The model under review builds one solid part; all positions refer to its coordinate system, in mm. Round coordinates to 2 decimals unless told otherwise and drop trailing zeros. Write each loop counter-clockwise with the first axis right and the second up, starting at its lowest first coordinate (ties: lowest second). Pieces come first, ordered by that corner, then holes. Notation, with made-up numbers: (48, -2.75) - (74, -2.75) arc R27 cw to (74, 21.25) - close; hole circle Ø4 at (46.25, -12). An arc over 180 degrees is marked (long way). Use one line per item in the form item = value.
from build123d import *

# Parameters (mm, degrees)
BOSS_EXTRUDE1_DEPTH = 2590.8
CUT_EXTRUDE1_DEPTH  = 2591.8
BOSS_EXTRUDE2_DEPTH = 2590.8
FILLET1_R           = 0.508


with BuildPart() as part:
    # Sketch1 → Boss-Extrude1 (new body)
    with BuildSketch(Plane(origin=(0, 0, 0), x_dir=(1, 0, 0), z_dir=(0, 1, 0))):
        with BuildLine():
            Line((101.58476, 5.338063609), (101.58476, 6.354063609))
            ThreePointArc((101.58476, 6.354063609), (50.79238, 19.05), (0, 6.354063609))
            Line((0, 6.354063609), (0, 5.338063609))
            Line((0, 5.338063609), (1.338554634, 5.338063609))
            ThreePointArc((1.338554634, 5.338063609), (45.188812602, 17.378377427), (90.062082389, 10.016044959))
            ThreePointArc((90.062082389, 10.016044959), (91.218156641, 9.549225792), (92.368682931, 9.068895628))
            ThreePointArc((92.368682931, 9.068895628), (96.251044015, 7.328911154), (100.06076, 5.435148318))
            Line((100.06076, 5.435148318), (100.06076, 4.322063609))
            ThreePointArc((100.06076, 4.322063609), (100.209549755, 3.962853364), (100.56876, 3.814063609))
            Line((100.56876, 3.814063609), (100.82276, 3.814063609))
            Line((100.82276, 3.814063609), (101.58476, 5.338063609))
        make_face()
    extrude(amount=BOSS_EXTRUDE1_DEPTH)

    # Sketch3 → Cut-Extrude1 (cut, through all)
    with BuildSketch(Plane(origin=(0, 2590.8, 0), x_dir=(1, 0, 0), z_dir=(0, 1, 0))):
        Polygon((100.06076, 2.923708758), (101.58476, 2.923708758), (101.58476, 5.592063609), (100.06076, 5.435148318), align=None)
        Polygon((0, 5.592063609), (0.4067845, 4.474432381), (0, 4.474432381), align=None)
    extrude(amount=-CUT_EXTRUDE1_DEPTH, mode=Mode.SUBTRACT)

    # Sketch2 → Boss-Extrude2 (add)
    with BuildSketch(Plane(origin=(0, 2590.8, 0), x_dir=(1, 0, 0), z_dir=(0, 1, 0))):
        with BuildLine():
            Line((101.238078351, 4.639563606), (101.58476, 5.592063609))
            Line((101.58476, 5.592063609), (97.711183428, 6.625490634))
            ThreePointArc((97.711183428, 6.625490634), (97.924124129, 6.275131553), (97.695976798, 5.934479203))
            ThreePointArc((97.695976798, 5.934479203), (96.254692814, 2.421137976), (99.718733273, 0.865088556))
            ThreePointArc((99.718733273, 0.865088556), (99.858345852, 0.953692868), (99.947271519, 1.093100982))
            Line((99.947271519, 1.093100982), (100.173716674, 1.715253931))
            ThreePointArc((100.173716674, 1.715253931), (100.127790714, 2.064096228), (99.815693785, 2.226563606))
            Line((99.815693785, 2.226563606), (98.79076, 2.226563606))
            ThreePointArc((98.79076, 2.226563606), (97.58426, 3.433063606), (98.79076, 4.639563606))
            Line((98.79076, 4.639563606), (101.238078351, 4.639563606))
        make_face()
        with BuildLine():
            ThreePointArc((1.769066215, 2.226563606), (1.456969286, 2.064096228), (1.411043326, 1.715253931))
            Line((1.411043326, 1.715253931), (1.637488481, 1.093100982))
            ThreePointArc((1.637488481, 1.093100982), (1.726414148, 0.953692868), (1.866026727, 0.865088556))
            ThreePointArc((1.866026727, 0.865088556), (5.330067186, 2.421137976), (3.888783202, 5.934479203))
            ThreePointArc((3.888783202, 5.934479203), (3.660635871, 6.275131553), (3.873576572, 6.625490634))
            Line((3.873576572, 6.625490634), (0, 5.592063609))
            Line((0, 5.592063609), (0.346681649, 4.639563606))
            Line((0.346681649, 4.639563606), (2.794, 4.639563606))
            ThreePointArc((2.794, 4.639563606), (4.0005, 3.433063606), (2.794, 2.226563606))
            Line((2.794, 2.226563606), (1.769066215, 2.226563606))
        make_face()
    extrude(amount=-BOSS_EXTRUDE2_DEPTH)

    # Fillet1
    fillet1_edges = [part.edges().sort_by_distance(p)[0] for p in [
        (101.238078351, 1295.4, -4.639563606),
        (0.346681649, 1295.4, -4.639563606),
    ]]
    fillet(fillet1_edges, radius=FILLET1_R)


solid = part.part
(1) To check wall thickness, follow L1, parallel to X at y = 232.5, z = -6.5; L2, parallel to X at y = 1887, z = -3.75; L3, parallel to Z at x = 46, y = 1734.5. State the ranges of each line that lie inside material, in increasing order.
Geometry results:
L1 = 0.27 to 3.73, 97.86 to 101.31
L2 = 3.96 to 5.51, 96.08 to 97.63
L3 = -18.94 to -17.42
(2) Add section B-B on z = -14. Write out the cut boundary in (x, y), then the cut area to 3 significant figures.
Geometry results:
outline = (18.16, 0) - (23.62, 0) - (23.62, 2590.8) - (18.16, 2590.8) - close; (77.96, 0) - (83.42, 0) - (83.42, 2590.8) - (77.96, 2590.8) - close
area = 28,300 mm2
(3) Add section A-A on y = 2063.5. Write out the cut boundary in (x, z).
Geometry results:
outline = (0, -6.35) arc R107.95 ccw to (101.58, -6.35) - (101.58, -5.59) - (101.36, -4.97) arc R0.51 ccw to (100.88, -4.64) - (98.79, -4.64) arc R1.21 cw to (98.79, -2.23) - (99.82, -2.23) arc R0.38 ccw to (100.17, -1.72) - (99.95, -1.09) arc R0.38 ccw to (99.72, -0.87) arc R2.73 ccw to (97.7, -5.93) arc R0.38 cw to (97.71, -6.63) arc R106.43 cw to (92.37, -9.07) arc R106.43 cw to (90.06, -10.02) arc R106.43 cw to (3.87, -6.63) arc R0.38 cw to (3.89, -5.93) arc R2.73 ccw to (1.87, -0.87) arc R0.38 ccw to (1.64, -1.09) - (1.41, -1.72) arc R0.38 ccw to (1.77, -2.23) - (2.79, -2.23) arc R1.21 cw to (2.79, -4.64) - (0.7, -4.64) arc R0.51 ccw to (0.23, -4.97) - (0, -5.59) - close
(4) Insertion check: P1, Ø1, axis at x = 100, y = 1770.5, coming from the +Z side; P2, Ø3, axis at x = 16.5, y = 798, coming from the -Z side; P3, Ø8, axis at x = 27.5, y = 426, coming from the -Z side. Each pin has a flat end and moves straight along its axis. Give the tip position at first contact, or say it passes through.
Geometry results:
P1 = -0.8
P2 = -13.95
P3 = -17.31
